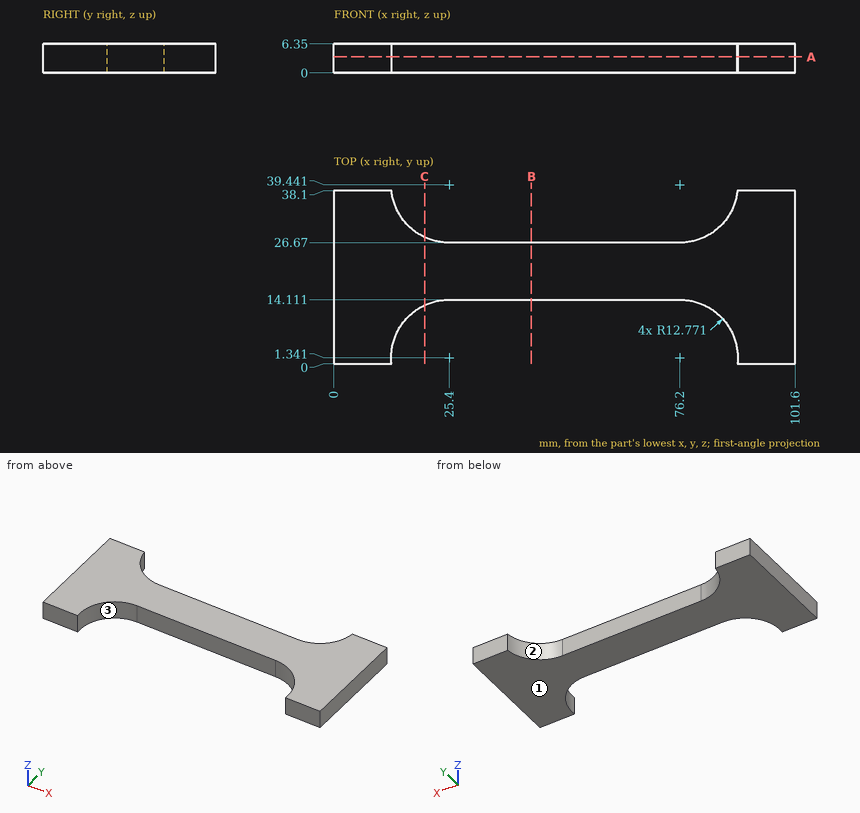
For this review, use the dimensioned drawing (mm, ordinates from the lowest corner) and the shaded views. Coordinates: 2 decimals unless noted, no trailing zeros. Loops run counter-clockwise (first coordinate to the right, second up) from the corner with the lowest first, then second, coordinate; pieces in that order, holes last. Notation, with made-up numbers: (-39.5, -37.75) -> (6.5, -37.75) arc R27 cw to (6.5, -4.75) -> close; hole circle Ø8 at (53.25, 75). An arc over 180 degrees is marked (long way). Use a Markdown table: item, result. Add a question column.
Item 1: Clearance check with flat-ended pins moving along their axes: P1, Ø1, axis at x = 45, z = 5, coming from the +Y side; P2, Ø3, axis at x = 23, z = 3, coming from the +Y side; P3, Ø1, axis at x = 34.5, z = 1, coming from the -Y side. State where each tip first meets the part, or that it passes through.
Item 2: The part is to be moulded in two halves that separate along X. For the marked faces 1, 2 and 3, say which applies: +X half, -X half, draft (parallel to the pull), parting line (faces both ways), or undercut.
Item 3: Wall thickness on L1, parallel to Y at x = 45.5, z = 4; L2, parallel to X at y = 34, z = 1.5 (1 decimal); L3, parallel to X at y = 36, z = 2.25: over which ranges is each line inside the solid? List them lowest first. Write a range as from..to.
Item 4: We need section B-B, the plane x = 43.5. Write out the cut boundary in (y, z).
Item 5: We need section C-C, the plane x = 20. Write out the cut boundary in (y, z).
Item 6: We need section A-A, the plane z = 3.5. Write out the cut boundary in (x, y), and give its area (3 significant figures).
Numbers:
| question | item | result |
|---|---|---|
| 1 | P1 | stops at y = 26.67 |
| 1 | P2 | stops at y = 27.28 |
| 1 | P3 | stops at y = 14.11 |
| 2 | face 1 | draft |
| 2 | face 2 | undercut |
| 2 | face 3 | undercut |
| 3 | L1 | y = 14.11..26.67 |
| 3 | L2 | x = 0..13.8, 87.8..101.6 |
| 3 | L3 | x = 0..13.1, 88.5..101.6 |
| 4 | outline | (14.11, 0) -> (26.67, 0) -> (26.67, 6.35) -> (14.11, 6.35) -> close |
| 5 | outline | (12.91, 0) -> (27.87, 0) -> (27.87, 6.35) -> (12.91, 6.35) -> close |
| 6 | outline | (0, 0) -> (12.7, 0) arc R12.77 cw to (25.4, 14.11) -> (76.2, 14.11) arc R12.77 cw to (88.9, 0) -> (101.6, 0) -> (101.6, 38.1) -> (88.9, 38.1) arc R12.77 cw to (76.2, 26.67) -> (25.4, 26.67) arc R12.77 cw to (12.7, 38.1) -> (0, 38.1) -> close |
| 6 | area | 2,060 mm^2 |
